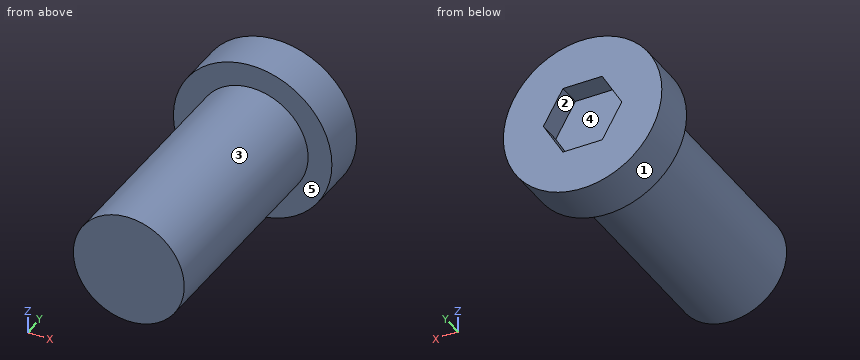
Autodesk Inventor part; units mm, degrees
ref_plane "YZ Plane" through (0, 0, 0) normal (1, 0, 0) x (0, 1, 0)
ref_plane "XZ Plane" through (0, 0, 0) normal (0, 1, 0) x (-1, 0, 0)
ref_plane "XY Plane" through (0, 0, 0) normal (0, 0, 1) x (1, 0, 0)
sketch "Sketch1" plane through (0, 0, 0) normal (0, 1, 0) x (-1, 0, 0)
  circle A0 centre (0, 0) radius 2.45
  dimension "d0" = 4.9
extrude "Extrusion1" add sketch "Sketch1" along normal blind 10
sketch "Sketch2" plane through (0, 10, 0) normal (0, 1, 0) x (1, 0, 0)
  circle A0 centre (0, 0) radius 3.5
  dimension "d3" = 7
extrude "Extrusion2" add sketch "Sketch2" along normal blind 2
thread "Thread1"
sketch "Sketch3" plane through (0, 12, 0) normal (0, 1, 0) x (1, 0, 0)
  line L0 (0.866, 1.5) -> (1.7321, 0)
  line L1 (1.7321, 0) -> (0.866, -1.5)
  line L2 (0.866, -1.5) -> (-0.866, -1.5)
  line L3 (-0.866, -1.5) -> (-1.7321, 0)
  line L4 (-1.7321, 0) -> (-0.866, 1.5)
  line L5 (-0.866, 1.5) -> (0.866, 1.5)
  point P0 (0, 0)
  point P1 (0, 0)
  dimension "d8" = 3
extrude "Extrusion3" cut sketch "Sketch3" against normal blind 1
equation "\"BendRadius\" = Thickness"
equation "\"BendReliefWidth\" = Thickness"
equation "\"BendReliefDepth\" = 0.5 * Thickness"
equation "\"CornerReliefSize\" = 4 * Thickness"
equation "\"MinimumRemnant\" = 2 * Thickness"
equation "\"TransitionRadius\" = BendRadius"
equation "\"JacobiRadiusSize\" = BendRadius"
equation "\"GapSize\" = Thickness"
properties part number "perno_simple"
The listing builds one solid part. Answer for the finished solid, in the listing's coordinates (mm). Face numbers are marked on the shaded views. A direction names the side the tool comes from. Round coordinates to 2 decimals unless told otherwise and drop trailing zeros. Order: outer loops, then holes, each group sorted by start corner. A loop starts at its lowest first (then second) coordinate and runs counter-clockwise, first axis right, second up. Notation, with made-up numbers: M 48,46 L 75,46 A13 cw 75,65 Z; hole C 28.25,-28.75 d11. An arc over 180 degrees is marked long. Answer in a Markdown table with one row per item. Add a question column.
1) Which of the six approach directions +Z, -Z, +X, -X, +Y, -Y give full straight-line access (tool end or side, diameter ignored) to the marked faces 1 and 2?
2) The part is cut by section C-C on y = 10.5. Determine the outline of the cut face in (x, z).
3) The part is cut by section B-B on z = 0.5. Determine the outline of the cut face in (x, y), plus the area to 3 significant figures.
4) Flat-ended cylindrical pins translate along their axes: pin 1 Ø2 at (x, y) = (1.5, 10) entering from -Z; pin 2 Ø3 at (y, z) = (10, -2) entering from -X; pin 3 Ø1.5 at (x, y) = (1.5, 10) entering from +Z. Find the tip coordinate at first contact, or state that the pin passes through.
5) Determine the mould class of the marked faces 3, 4 and 5 for opening direction X: pulls with the +X half, pulls with the -X half, needs draft (parallel to the pull), parting line crosses it, or undercut.
6) The part is cut by section D-D on x = 2. Determine the outline of the cut face in (y, z).
7) The part is cut by section A-A on x = 0. Determine the outline of the cut face in (y, z).
8) Consider line 1 along Y through (x, z) = (-2.5, 1); line 2 along Y through (x, z) = (0.5, -0.5); line 3 along X through (y, z) = (11.25, -2). Determine where each line is inside the solid, lowest interval first. Write a range as from..to.
Findings below:
| question | item | result |
|---|---|---|
| 1 | face 1 | +Y, -Y |
| 1 | face 2 | +Y |
| 2 | outline | C 0,0 d7 |
| 3 | outline | M -3.46,10 L -2.4,10 L -2.4,0 L 2.4,0 L 2.4,10 L 3.46,10 L 3.46,12 L 1.44,12 L 1.44,11 L -1.44,11 L -1.44,12 L -3.46,12 Z |
| 3 | area | 58.9 mm² |
| 4 | pin 1 | stops at z = -3.46 |
| 4 | pin 2 | stops at x = -3.46 |
| 4 | pin 3 | stops at z = 3.42 |
| 5 | face 3 | parting line crosses it |
| 5 | face 4 | undercut |
| 5 | face 5 | needs draft |
| 6 | outline | M 0,-1.42 L 10,-1.42 L 10,-2.87 L 12,-2.87 L 12,2.87 L 10,2.87 L 10,1.42 L 0,1.42 Z |
| 7 | outline | M 0,-2.45 L 10,-2.45 L 10,-3.5 L 12,-3.5 L 12,-1.5 L 11,-1.5 L 11,1.5 L 12,1.5 L 12,3.5 L 10,3.5 L 10,2.45 L 0,2.45 Z |
| 8 | line 1 | y = 10..12 |
| 8 | line 2 | y = 0..11 |
| 8 | line 3 | x = -2.87..2.87 |
